Autodesk Inventor part; units mm, degrees
ref_plane "YZ Plane" through (0, 0, 0) normal (1, 0, 0) x (0, 1, 0)
ref_plane "XZ Plane" through (0, 0, 0) normal (0, 1, 0) x (-1, 0, 0)
ref_plane "XY Plane" through (0, 0, 0) normal (0, 0, 1) x (1, 0, 0)
sketch "Sketch1" plane through (0, 0, 0) normal (0, 0, 1) x (1, 0, 0)
  line L0 (0, 4.2) -> (0, -4.2)
  line L1 (-4.8497, 0) -> (4.8497, 0)
  line L2 (-3.4641, 0) -> (-1.7321, 3)
  line L3 (-1.7321, 3) -> (1.7321, 3)
  line L4 (1.7321, 3) -> (3.4641, 0)
  line L5 (3.4641, 0) -> (1.7321, -3)
  line L6 (1.7321, -3) -> (-1.7321, -3)
  line L7 (-1.7321, -3) -> (-3.4641, 0)
  point P0 (0, 0)
  dimension "d0" = 6
extrude "Extrusion1" add sketch "Sketch1" along normal blind 10
sketch "Sketch2" plane through (0, 0, 10) normal (0, 0, 1) x (1, 0, 0)
  point P0 (0, 0)
  point P1 (0, 0)
hole "Hole1" at (0, 0, 10) direction (0, 0, -1) diameter 2.459 depth 6 tip angle 118
sketch "Sketch3" plane through (0, 0, 0) normal (0, 0, -1) x (-1, 0, 0)
  circle A0 centre (0, 0) radius 1.5
  dimension "d10" = 3
extrude "Extrusion2" add sketch "Sketch3" along normal blind 5
chamfer "Chamfer1" distance 0.5 angle 45 1 edges at (1.5, 0, -5)
thread "Thread1"
properties part number "Entretoise Hex 6 x 10"
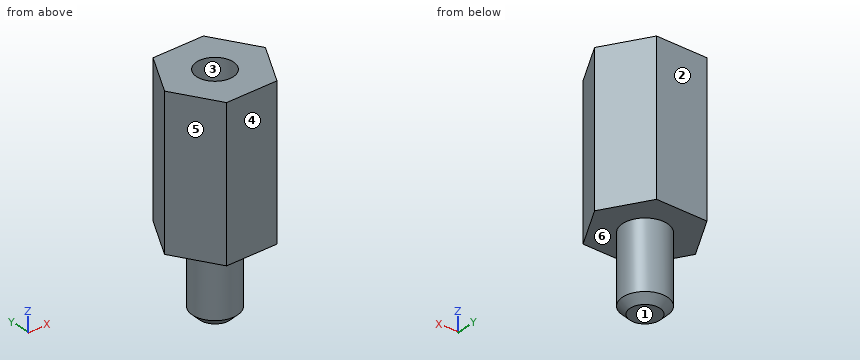
Work out the finished part from the listing and answer in its coordinate system (mm). Face numbers are marked on the shaded views. A direction names the side the tool comes from. Round coordinates to 2 decimals unless told otherwise and drop trailing zeros. Order: outer loops, then holes, each group sorted by start corner. A loop starts at its lowest first (then second) coordinate and runs counter-clockwise, first axis right, second up.
Q1. A cutting plane is placed at D-D, the plane y = 2. Determine the outline of the cut face in (x, z).
Solution:
outline: (-2.31, 0) - (2.31, 0) - (2.31, 10) - (-2.31, 10) - close
Q2. The mould has two halves that part along Y. Classify the marked faces 1, 2, 3 and 4: pulls with the +Y half, pulls with the -Y half, needs draft (parallel to the pull), parting line crosses it, or undercut.
Solution:
face 1: needs draft
face 2: pulls with the +Y half
face 3: undercut
face 4: pulls with the -Y half
Q3. A tool of negligible diameter and unlimited length cuts with its end or side. For the marked faces 5 and 6, from which of +Z, -Z, +X, -X, +Y, -Y can it reach the whole face along a straight path? Write none if from no direction.
Solution:
face 5: +Z, -Z, -X, -Y
face 6: -Z
Q4. Given pin 1 Ø1.5 at (x, y) = (-2.5, 0.5) entering from -Z; pin 2 Ø3 at (x, z) = (-2, -0.5) entering from +Y, each flat-ended and moving along its own axis, determine where each tip first touches the part or whether it passes through.
Solution:
pin 1: stops at z = 0
pin 2: stops at y = 3
Q5. Find the intervals of material crossed by line 1 along Y through (x, z) = (0, 5.55); line 2 along Z through (x, y) = (2.25, 1.7); line 3 along X through (y, z) = (0.1, -3.75), in increasing order.
Solution:
line 1: y = -3 to -1.23, 1.23 to 3
line 2: z = 0 to 10
line 3: x = -1.5 to 1.5
Q6. A cutting plane is placed at A-A, the plane z = 7.25. Determine the outline of the cut face in (x, y).
Solution:
outline: (-3.46, 0) - (-1.73, -3) - (1.73, -3) - (3.46, 0) - (1.73, 3) - (-1.73, 3) - close; hole circle Ø2.46 at (0, 0)
Q7. A cutting plane is placed at B-B, the plane z = 3. Determine the outline of the cut face in (x, y), then the cut area to 3 significant figures.
Solution:
outline: (-3.46, 0) - (-1.73, -3) - (1.73, -3) - (3.46, 0) - (1.73, 3) - (-1.73, 3) - close
area: 31.2 mm2
Q8. A cutting plane is placed at C-C, the plane x = -2. Determine the outline of the cut face in (y, z).
Solution:
outline: (-2.54, 0) - (2.54, 0) - (2.54, 10) - (-2.54, 10) - close
